Model file for the job. Use its own axes, mm. Face numbers are marked on the shaded views. A direction names the side the tool comes from. Round coordinates to 2 decimals unless told otherwise and drop trailing zeros. Loops run counter-clockwise (first coordinate to the right, second up) from the corner with the lowest first, then second, coordinate; pieces in that order, holes last. Notation, with made-up numbers: (35, 81.25) -> (85, 81.25) arc R21 ccw to (85, 88.25) -> close; hole circle Ø5 at (-6.75, 77). An arc over 180 degrees is marked (long way). Use a Markdown table: item, result.
from build123d import *

# Parameters (mm, degrees)
SKETCH1_W           = 4.572
SKETCH1_H           = 5.334
BOSS_EXTRUDE1_DEPTH = 5.334


with BuildPart() as part:
    # Sketch1 → Boss-Extrude1 (new body)
    with BuildSketch(Plane(origin=(0, 0, 0), x_dir=(0, 0, -1), z_dir=(1, 0, 0))):
        Polygon((-15.875, -29.21), (-1.5, -29.21), (-1.5, -20.71), (-2.75, -20.71), (-2.75, -18.51), (2.75, -18.51), (2.75, -20.71), (1.5, -20.71), (1.5, -29.21), (15.875, -29.21), (15.875, 29.21), (10.922, 29.21), (10.922, 34.544), (6.35, 34.544), (6.35, 29.21), (1.5, 29.21), (1.5, 20.71), (2.75, 20.71), (2.75, 18.51), (-2.75, 18.51), (-2.75, 20.71), (-1.5, 20.71), (-1.5, 29.21), (-6.35, 29.21), (-6.35, 34.544), (-10.922, 34.544), (-10.922, 29.21), (-15.875, 29.21), align=None)
        with Locations((-8.636, -31.877)):
            Rectangle(SKETCH1_W, SKETCH1_H)
        with Locations((8.636, -31.877)):
            Rectangle(SKETCH1_W, SKETCH1_H)
    extrude(amount=BOSS_EXTRUDE1_DEPTH)


solid = part.part
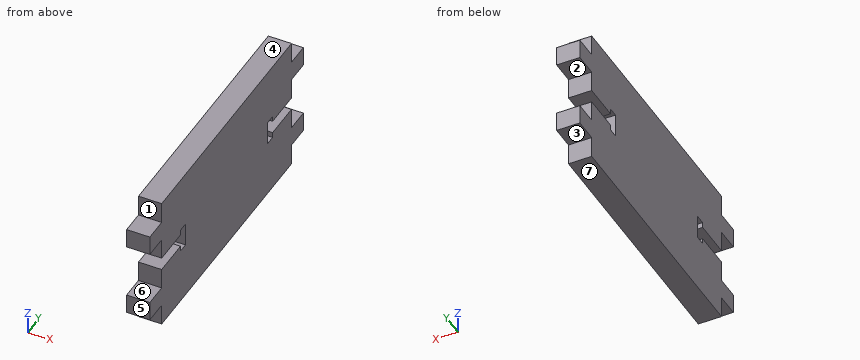
Q1. Band-saw the part on A-A, the plane y = 22. Give the cut face in (x, z) (3 decimals).
Results list:
| item | result |
|---|---|
| outline | (0, -15.875) -> (5.334, -15.875) -> (5.334, -1.5) -> (0, -1.5) -> close; (0, 1.5) -> (5.334, 1.5) -> (5.334, 15.875) -> (0, 15.875) -> close |
Q2. Drill centre lines: L1, parallel to Y at x = 3.4, z = -2.5; L2, parallel to Z at x = 3.6, y = -28 (3 decimals); L3, parallel to Y at x = 3.45, z = -14. Where is each one in solid material? Low to high. Write a range as from..to.
Results list:
| item | result |
|---|---|
| L1 | y = -29.21..-20.71, -18.51..18.51, 20.71..29.21 |
| L2 | z = -15.875..-1.5, 1.5..15.875 |
| L3 | y = -29.21..29.21 |
Q3. Tool access for the marked faces 1, 2 and 3: list every direction of +Z, -Z, +X, -X, +Y, -Y with a clear straight run to the whole face (end or side of a thin tool).
Results list:
| item | result |
|---|---|
| face 1 | +Z, +X, -X, -Y |
| face 2 | +X, -X, +Y |
| face 3 | -Z, +X, -X, +Y |
Q4. Pull direction Z, two halves, no side cores. Call the marked faces 4, 5, 6 and 7: released by +Z, released by -Z, zero draft, split by the parting line, or undercut.
Results list:
| item | result |
|---|---|
| face 4 | released by +Z |
| face 5 | zero draft |
| face 6 | undercut |
| face 7 | released by -Z |
Q5. Band-saw the part on B-B, the plane z = 4. Give the cut face in (x, y).
Results list:
| item | result |
|---|---|
| outline | (0, -29.21) -> (5.33, -29.21) -> (5.33, 29.21) -> (0, 29.21) -> close |
Q6. Flat gauge pins, fed straight in: pin 1 (2.5 mm diameter, centred on x = 2, z = -13, fed in from -Y); pin 2 (1.6 mm diameter, centred on x = 3, y = -32.5, fed in from +Z); pin 3 (0.6 mm diameter, centred on x = 2, z = 2, fed in from +Y). Where does each tip first touch, or does it go through?
Results list:
| item | result |
|---|---|
| pin 1 | stops at y = -29.21 |
| pin 2 | stops at z = 10.92 |
| pin 3 | stops at y = 29.21 |
